Design review of the part built by this model. Coordinates are the model's own, in mm. Face numbers are marked on the shaded views. Round coordinates to 2 decimals unless told otherwise and drop trailing zeros. Loops run counter-clockwise (first coordinate to the right, second up) from the corner with the lowest first, then second, coordinate; pieces in that order, holes last. Notation, with made-up numbers: (3.25, 64.25) -> (11.25, 64.25) arc R31 ccw to (11.25, 99.25) -> close; hole circle Ø5 at (84, -36.75). An arc over 180 degrees is marked (long way). Write each question's results on one line, items separated by ' | '. Start each with the question number.
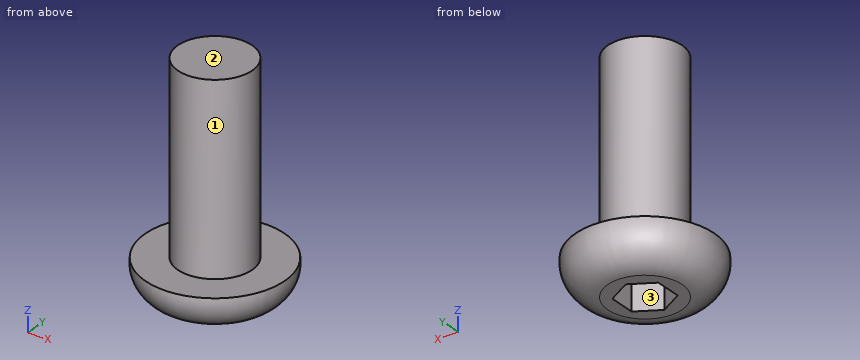
from build123d import *

# Parameters (mm, degrees)
CUT_EXTRUDE1_DEPTH = 1.8


with BuildPart() as part:
    # Sketch1 → Revolve1 (revolve)
    with BuildSketch(Plane(origin=(0, 0, 0), x_dir=(1, 0, 0), z_dir=(0, 1, 0))):
        with BuildLine():
            Line((0, 0), (-2, 0))
            Line((-2, 0), (-2, 10))
            Line((-2, 10), (-3.75, 10))
            ThreePointArc((-3.75, 10), (-3.328768227, 11.397047198), (-2, 12))
            Line((-2, 12), (0, 12))
            Line((0, 12), (0, 0))
        make_face()
    revolve(axis=Axis((0, 0, 0), (0, 0, -1)))

    # Sketch2 → Cut-Extrude1 (cut)
    with BuildSketch(Plane(origin=(0, 0, -12), x_dir=(-1, 0, 0), z_dir=(0, 0, -1))):
        Polygon((0, -1.443375673), (1.25, -0.721687836), (1.25, 0.721687836), (0, 1.443375673), (-1.25, 0.721687836), (-1.25, -0.721687836), align=None)
    extrude(amount=-CUT_EXTRUDE1_DEPTH, mode=Mode.SUBTRACT)


solid = part.part
1) The part is to be moulded in two halves that separate along Y. For the marked faces 1, 2 and 3, say which applies: +Y half, -Y half, draft (parallel to the pull), parting line (faces both ways), or undercut.
2) To check wall thickness, follow line 1 (Z direction, x = 0, y = 0.25); line 2 (X direction, y = -1, z = -10.75); line 3 (Z direction, x = -1.75, y = 3). State the ranges of each line that lie inside material, in increasing order. Write a range as from..to.
3) Insertion check: pin 1 (4 mm diameter, centred on x = 0.5, y = -1, fed in from -Z); pin 2 (4 mm diameter, centred on x = -1, z = -5, fed in from -Y); pin 3 (1 mm diameter, centred on x = 0, y = 0.5, fed in from -Z); pin 4 (2 mm diameter, centred on y = -2, z = -6, fed in from +X). Each pin has a flat end and moves straight along its axis. Give the tip position at first contact, or say it passes through.
4) Take a section at A-A (z = -3.25). Write out the cut boundary in (x, y), plus the area to 3 significant figures.
Geometry check:
1) face 1: parting line | face 2: draft | face 3: undercut
2) line 1: z = -10.2..0 | line 2: x = -3.55..-0.77, 0.77..3.55 | line 3: z = -11.21..-10
3) pin 1: stops at z = -12 | pin 2: stops at y = -2 | pin 3: stops at z = -10.2 | pin 4: stops at x = 1.73
4) outline: circle Ø4 at (0, 0) | area: 12.6 mm^2
